The listing builds one solid part. Answer for the finished solid, in the listing's coordinates (mm). A direction names the side the tool comes from. Round coordinates to 2 decimals unless told otherwise and drop trailing zeros. Write each loop counter-clockwise with the first axis right and the second up, starting at its lowest first coordinate (ties: lowest second). Pieces come first, ordered by that corner, then holes. Notation, with made-up numbers: (63, -15) -> (104, -15) arc R12 cw to (104, 3) -> close; hole circle Ø9 at (-4.75, 60.25). An arc over 180 degrees is marked (long way). Write each question's results on one line, items separated by ' | '. Start each with the question number.
```python
from build123d import *

# Parameters (mm, degrees)
SKETCH2_W                      = 3.9
SKETCH2_H                      = 3.9
F_40_SERIES_TS40_120LM_1_DEPTH = 380
M8X1_25_TAPPED_HOLE1_D         = 6.8
M8X1_25_TAPPED_HOLE1_DEPTH     = 30
M8X1_25_TAPPED_HOLE1_TIP       = 2.042926105
M8X1_25_TAPPED_HOLE2_D         = 6.8
M8X1_25_TAPPED_HOLE2_DEPTH     = 30
M8X1_25_TAPPED_HOLE2_TIP       = 2.042926105


with BuildPart() as part:
    # Sketch2 → 40 series TS40-120LM(1) (new body)
    with BuildSketch(Plane.XY.offset(-190)):
        with BuildLine():
            Line((15.3, -35.9), (20, -35.9))
            Line((20, -35.9), (20, -4.1))
            Line((20, -4.1), (15.3, -4.1))
            Line((15.3, -4.1), (15.3, -7.6))
            Line((15.3, -7.6), (17.65, -7.6))
            Line((17.65, -7.6), (17.65, -10.1))
            Line((17.65, -10.1), (13.6, -10.1))
            Line((13.6, -10.1), (7.6, -4.1))
            Line((7.6, -4.1), (7.6, 4.1))
            Line((7.6, 4.1), (13.6, 10.1))
            Line((13.6, 10.1), (17.65, 10.1))
            Line((17.65, 10.1), (17.65, 7.6))
            Line((17.65, 7.6), (15.3, 7.6))
            Line((15.3, 7.6), (15.3, 4.1))
            Line((15.3, 4.1), (20, 4.1))
            Line((20, 4.1), (20, 35.9))
            Line((20, 35.9), (15.3, 35.9))
            Line((15.3, 35.9), (15.3, 32.4))
            Line((15.3, 32.4), (17.65, 32.4))
            Line((17.65, 32.4), (17.65, 29.9))
            Line((17.65, 29.9), (13.6, 29.9))
            Line((13.6, 29.9), (7.6, 35.9))
            Line((7.6, 35.9), (7.6, 44.1))
            Line((7.6, 44.1), (13.6, 50.1))
            Line((13.6, 50.1), (17.65, 50.1))
            Line((17.65, 50.1), (17.65, 47.6))
            Line((17.65, 47.6), (15.3, 47.6))
            Line((15.3, 47.6), (15.3, 44.1))
            Line((15.3, 44.1), (20, 44.1))
            Line((20, 44.1), (20, 57.5))
            ThreePointArc((20, 57.5), (19.267766953, 59.267766953), (17.5, 60))
            Line((17.5, 60), (4.1, 60))
            Line((4.1, 60), (4.1, 55.3))
            Line((4.1, 55.3), (7.6, 55.3))
            Line((7.6, 55.3), (7.6, 57.65))
            Line((7.6, 57.65), (10.1, 57.65))
            Line((10.1, 57.65), (10.1, 53.6))
            Line((10.1, 53.6), (4.1, 47.6))
            Line((4.1, 47.6), (-4.1, 47.6))
            Line((-4.1, 47.6), (-10.1, 53.6))
            Line((-10.1, 53.6), (-10.1, 57.65))
            Line((-10.1, 57.65), (-7.6, 57.65))
            Line((-7.6, 57.65), (-7.6, 55.3))
            Line((-7.6, 55.3), (-4.1, 55.3))
            Line((-4.1, 55.3), (-4.1, 60))
            Line((-4.1, 60), (-17.5, 60))
            ThreePointArc((-17.5, 60), (-19.267766953, 59.267766953), (-20, 57.5))
            Line((-20, 57.5), (-20, 44.1))
            Line((-20, 44.1), (-15.3, 44.1))
            Line((-15.3, 44.1), (-15.3, 47.6))
            Line((-15.3, 47.6), (-17.65, 47.6))
            Line((-17.65, 47.6), (-17.65, 50.1))
            Line((-17.65, 50.1), (-13.6, 50.1))
            Line((-13.6, 50.1), (-7.6, 44.1))
            Line((-7.6, 44.1), (-7.6, 35.9))
            Line((-7.6, 35.9), (-13.6, 29.9))
            Line((-13.6, 29.9), (-17.65, 29.9))
            Line((-17.65, 29.9), (-17.65, 32.4))
            Line((-17.65, 32.4), (-15.3, 32.4))
            Line((-15.3, 32.4), (-15.3, 35.9))
            Line((-15.3, 35.9), (-20, 35.9))
            Line((-20, 35.9), (-20, 4.1))
            Line((-20, 4.1), (-15.3, 4.1))
            Line((-15.3, 4.1), (-15.3, 7.6))
            Line((-15.3, 7.6), (-17.65, 7.6))
            Line((-17.65, 7.6), (-17.65, 10.1))
            Line((-17.65, 10.1), (-13.6, 10.1))
            Line((-13.6, 10.1), (-7.6, 4.1))
            Line((-7.6, 4.1), (-7.6, -4.1))
            Line((-7.6, -4.1), (-13.6, -10.1))
            Line((-13.6, -10.1), (-17.65, -10.1))
            Line((-17.65, -10.1), (-17.65, -7.6))
            Line((-17.65, -7.6), (-15.3, -7.6))
            Line((-15.3, -7.6), (-15.3, -4.1))
            Line((-15.3, -4.1), (-20, -4.1))
            Line((-20, -4.1), (-20, -35.9))
            Line((-20, -35.9), (-15.3, -35.9))
            Line((-15.3, -35.9), (-15.3, -32.4))
            Line((-15.3, -32.4), (-17.65, -32.4))
            Line((-17.65, -32.4), (-17.65, -29.9))
            Line((-17.65, -29.9), (-13.6, -29.9))
            Line((-13.6, -29.9), (-7.6, -35.9))
            Line((-7.6, -35.9), (-7.6, -44.1))
            Line((-7.6, -44.1), (-13.6, -50.1))
            Line((-13.6, -50.1), (-17.65, -50.1))
            Line((-17.65, -50.1), (-17.65, -47.6))
            Line((-17.65, -47.6), (-15.3, -47.6))
            Line((-15.3, -47.6), (-15.3, -44.1))
            Line((-15.3, -44.1), (-20, -44.1))
            Line((-20, -44.1), (-20, -57.5))
            ThreePointArc((-20, -57.5), (-19.267766953, -59.267766953), (-17.5, -60))
            Line((-17.5, -60), (-4.1, -60))
            Line((-4.1, -60), (-4.1, -55.3))
            Line((-4.1, -55.3), (-7.6, -55.3))
            Line((-7.6, -55.3), (-7.6, -57.65))
            Line((-7.6, -57.65), (-10.1, -57.65))
            Line((-10.1, -57.65), (-10.1, -53.6))
            Line((-10.1, -53.6), (-4.1, -47.6))
            Line((-4.1, -47.6), (4.1, -47.6))
            Line((4.1, -47.6), (10.1, -53.6))
            Line((10.1, -53.6), (10.1, -57.65))
            Line((10.1, -57.65), (7.6, -57.65))
            Line((7.6, -57.65), (7.6, -55.3))
            Line((7.6, -55.3), (4.1, -55.3))
            Line((4.1, -55.3), (4.1, -60))
            Line((4.1, -60), (17.5, -60))
            ThreePointArc((17.5, -60), (19.267766953, -59.267766953), (20, -57.5))
            Line((20, -57.5), (20, -44.1))
            Line((20, -44.1), (15.3, -44.1))
            Line((15.3, -44.1), (15.3, -47.6))
            Line((15.3, -47.6), (17.65, -47.6))
            Line((17.65, -47.6), (17.65, -50.1))
            Line((17.65, -50.1), (13.6, -50.1))
            Line((13.6, -50.1), (7.6, -44.1))
            Line((7.6, -44.1), (7.6, -35.9))
            Line((7.6, -35.9), (13.6, -29.9))
            Line((13.6, -29.9), (17.65, -29.9))
            Line((17.65, -29.9), (17.65, -32.4))
            Line((17.65, -32.4), (15.3, -32.4))
            Line((15.3, -32.4), (15.3, -35.9))
        make_face()
        Polygon((-4.1, -7.6), (4.1, -7.6), (8.6, -12.1), (17.65, -12.1), (17.65, -27.9), (8.6, -27.9), (4.1, -32.4), (-4.1, -32.4), (-8.6, -27.9), (-17.65, -27.9), (-17.65, -12.1), (-8.6, -12.1), align=None, mode=Mode.SUBTRACT)
        Polygon((-4.1, 7.6), (-8.6, 12.1), (-17.65, 12.1), (-17.65, 27.9), (-8.6, 27.9), (-4.1, 32.4), (4.1, 32.4), (8.6, 27.9), (17.65, 27.9), (17.65, 12.1), (8.6, 12.1), (4.1, 7.6), align=None, mode=Mode.SUBTRACT)
        with Locations((15.55, -55.55)):
            Rectangle(SKETCH2_W, SKETCH2_H, mode=Mode.SUBTRACT)
        with Locations((-15.55, -55.55)):
            Rectangle(SKETCH2_W, SKETCH2_H, mode=Mode.SUBTRACT)
        with Locations((-15.55, 55.55)):
            Rectangle(SKETCH2_W, SKETCH2_H, mode=Mode.SUBTRACT)
        with Locations((15.55, 55.55)):
            Rectangle(SKETCH2_W, SKETCH2_H, mode=Mode.SUBTRACT)
        with BuildLine():
            ThreePointArc((0, -43.35), (3.35, -40), (0, -36.65))
            ThreePointArc((0, -36.65), (-3.35, -40), (0, -43.35))
        make_face(mode=Mode.SUBTRACT)
        with BuildLine():
            ThreePointArc((3.35, 0), (0, -3.35), (-3.35, 0))
            ThreePointArc((-3.35, 0), (0, 3.35), (3.35, 0))
        make_face(mode=Mode.SUBTRACT)
        with BuildLine():
            ThreePointArc((0, 43.35), (-3.35, 40), (0, 36.65))
            ThreePointArc((0, 36.65), (3.35, 40), (0, 43.35))
        make_face(mode=Mode.SUBTRACT)
    extrude(amount=F_40_SERIES_TS40_120LM_1_DEPTH)

    # M8x1.25 Tapped Hole1
    with Locations(Plane.XY.offset(190)):
        with Locations((0, 40), (0, 0), (0, -40)):
            Hole(M8X1_25_TAPPED_HOLE1_D / 2, depth=M8X1_25_TAPPED_HOLE1_DEPTH)
            with Locations((0, 0, -(M8X1_25_TAPPED_HOLE1_DEPTH + M8X1_25_TAPPED_HOLE1_TIP / 2))):  # 118° drill point
                Cone(0, M8X1_25_TAPPED_HOLE1_D / 2, M8X1_25_TAPPED_HOLE1_TIP, mode=Mode.SUBTRACT)

    # M8x1.25 Tapped Hole2
    with Locations(Plane(origin=(0, 0, -190), x_dir=(-1, 0, 0), z_dir=(0, 0, -1))):
        with Locations((0, 40), (0, 0)):
            Hole(M8X1_25_TAPPED_HOLE2_D / 2, depth=M8X1_25_TAPPED_HOLE2_DEPTH)
            with Locations((0, 0, -(M8X1_25_TAPPED_HOLE2_DEPTH + M8X1_25_TAPPED_HOLE2_TIP / 2))):  # 118° drill point
                Cone(0, M8X1_25_TAPPED_HOLE2_D / 2, M8X1_25_TAPPED_HOLE2_TIP, mode=Mode.SUBTRACT)


solid = part.part
```
Q1. Find the intervals of material crossed by line 1 (Y direction, x = 13, z = -44); line 2 (Y direction, x = -1, z = 45); line 3 (X direction, y = 13, z = 37), in increasing order.
Q2. The part is cut by section B-B, the plane y = -40. Write down the section's boundary in (x, z), then the cut area to 3 significant figures.
Q3. Determine the mould class of faces 1 (the flat face through (11, -60, -3)), 2 (the flat face through (20, -20, -3)), 3 (the cylindrical face through (-0.44, 43.37, -174.79)), 4 (the flat face through (-17.65, -20, -3)) for opening direction Y: pulls with the +Y half, pulls with the -Y half, needs draft (parallel to the pull), parting line crosses it, or undercut.
Q4. This flat-tipped pin is pushed along its axis until it touches: pin 1 (3 mm diameter, centred on y = -42.5, z = 72, fed in from +X). Where does it stop, or does it pass through?
Q5. The part is cut by section A-A, the plane y = 0. Write down the section's boundary in (x, z), then the cut area to 3 significant figures.
Q6. For faces 5 (the flat face through (11, 60, -3)), 6 (the flat face through (0, 47.6, -3)), 7 (the flat face through (-17.65, 20, -3)), 8 (the flat face through (-7.6, 0, -3)), determine the directions among +Z, -Z, +X, -X, +Y, -Y from which every point of the face is accessible in a straight line to the end or side of a thin tool.
Q7. The part is cut by section C-C, the plane z = -136.5. State how many separate pieces and enclosed holes the cut face has, then the cut area to 3 significant figures.
Answers follow:
1) line 1: -60 to -49.5, -30.5 to -27.9, -12.1 to -9.5, 9.5 to 12.1, 27.9 to 30.5, 49.5 to 60 | line 2: -47.6 to -43.2, -36.8 to -32.4, -7.6 to -3.2, 3.2 to 7.6, 32.4 to 36.8, 43.2 to 47.6 | line 3: -20 to -17.65, 17.65 to 20
2) outline: (-7.6, -190) -> (-3.35, -190) -> (-3.35, 159.97) -> (-3.4, 160) -> (-3.4, 190) -> (-7.6, 190) -> close; (3.35, -190) -> (7.6, -190) -> (7.6, 190) -> (3.4, 190) -> (3.4, 160) -> (3.35, 159.97) -> close | area: 3,230 mm^2
3) face 1: pulls with the -Y half | face 2: needs draft | face 3: undercut | face 4: undercut
4) pin 1: x = 7.6
5) outline: (-7.6, -190) -> (-3.4, -190) -> (-3.4, -160) -> (-3.35, -159.97) -> (-3.35, 159.97) -> (-3.4, 160) -> (-3.4, 190) -> (-7.6, 190) -> close; (3.35, -159.97) -> (3.4, -160) -> (3.4, -190) -> (7.6, -190) -> (7.6, 190) -> (3.4, 190) -> (3.4, 160) -> (3.35, 159.97) -> close | area: 3,220 mm^2
6) face 5: +Z, -Z, +X, -X, +Y | face 6: +Z, -Z, +Y | face 7: +Z, -Z | face 8: +Z, -Z, -X
7) separate pieces: 1 | enclosed holes: 9 | area: 1,930 mm^2
